```python
from build123d import *

# Parameters (mm, degrees)
SKETCH1_W           = 10
SKETCH1_H           = 5
BOSS_EXTRUDE1_DEPTH = 1
SKETCH1_3_W         = 10
SKETCH1_3_H         = 5
SKETCH1_3_W_2       = 8
SKETCH1_3_H_2       = 3
BOSS_EXTRUDE2_DEPTH = 1


with BuildPart() as part:
    # Sketch1 → Boss-Extrude1 (new body)
    with BuildSketch(Plane(origin=(0, 0, 0), x_dir=(1, 0, 0), z_dir=(0, 1, 0))):
        Rectangle(SKETCH1_W, SKETCH1_H)
    extrude(amount=BOSS_EXTRUDE1_DEPTH)

    # Sketch1_3 → Boss-Extrude2 (add)
    with BuildSketch(Plane(origin=(0, 0, 0), x_dir=(1, 0, 0), z_dir=(0, 1, 0))):
        Rectangle(SKETCH1_3_W, SKETCH1_3_H)
        Rectangle(SKETCH1_3_W_2, SKETCH1_3_H_2, mode=Mode.SUBTRACT)
    extrude(amount=-BOSS_EXTRUDE2_DEPTH)


solid = part.part
```
Input: part model. Units: mm. Frame: model coordinates. A direction names the side the tool comes from. Give positions to 0.01 mm unless a question says otherwise; leave off trailing zeros. Order: outer loops, then holes, each group sorted by start corner. A loop starts at its lowest first (then second) coordinate and runs counter-clockwise, first axis right, second up.
1. Material intervals for L1, parallel to X at y = -0.2, z = -1.4; L2, parallel to Z at x = -3.75, y = -0.3; L3, parallel to Y at x = -0.25, z = 0.05, sorted ascending.
Derived:
L1: x = -5 to -4, 4 to 5
L2: z = -2.5 to -1.5, 1.5 to 2.5
L3: y = 0 to 1
2. Section C-C on z = -0.2. Return the cut outline in (x, y).
Derived:
outline: (-5, -1) - (-4, -1) - (-4, 0) - (4, 0) - (4, -1) - (5, -1) - (5, 1) - (-5, 1) - close
3. Section A-A on y = -0.1. Return the cut outline in (x, z).
Derived:
outline: (-5, -2.5) - (5, -2.5) - (5, 2.5) - (-5, 2.5) - close; hole (-4, -1.5) - (4, -1.5) - (4, 1.5) - (-4, 1.5) - close
4. Section B-B on x = -1.75. Return the cut outline in (y, z), and give its area (3 significant figures).
Derived:
outline: (-1, -2.5) - (1, -2.5) - (1, 2.5) - (-1, 2.5) - (-1, 1.5) - (0, 1.5) - (0, -1.5) - (-1, -1.5) - close
area: 7.00 mm2
5. Mould query, pull axis Z, two halves, no side actions, for faces 1 (the flat face through (0, 0, 2.5)), 2 (the flat face through (0, 0, 0)), 3 (the flat face through (5, 0, 0)). Classes: released by +Z, released by -Z, zero draft, split by the parting line, or undercut.
Derived:
face 1: released by +Z
face 2: undercut
face 3: zero draft
6. Reachability of faces 4 (the flat face through (-0.1, -0.5, 1.5)), 5 (the flat face through (0, 0, -2.5)) from +Z, -Z, +X, -X, +Y, -Y: full face, straight path, thin tool, end or side. Return the list, or none.
Derived:
face 4: -Y
face 5: -Z, +X, -X, +Y, -Y
7. Pin query (flat end, axial travel): pin 1 (1.5 mm diameter, centred on x = -1, z = 0, fed in from -Y). Return the tip coordinate at first contact, or that it passes through.
Derived:
pin 1: stops at y = 0
